Geometry check sheet. Reference: the model listing, model coordinates, mm. Round coordinates to 2 decimals unless told otherwise and drop trailing zeros. Order: outer loops, then holes, each group sorted by start corner. A loop starts at its lowest first (then second) coordinate and runs counter-clockwise, first axis right, second up. Notation, with made-up numbers: (-0.5, 47.5) - (20.5, 47.5) arc R30 ccw to (20.5, 79.5) - close; hole circle Ø7 at (-24, 49). An arc over 180 degrees is marked (long way). Use a Markdown table: item, result. Add a question column.
(1) Section check C-C on y = 1.05. Record the boundary of the cut face in (x, z).
(2) Gauge pin test, flat ends, axial feed: P1, Ø4.5, axis at x = 7.5, z = -7.5, coming from the +Y side; P2, Ø4.5, axis at x = 7.5, z = -78.5, coming from the -Y side; P3, Ø4, axis at x = 48.5, z = -7.5, coming from the +Y side. Record the tip position at first contact, or that the pin passes through.
(3) Section check A-A on x = 7.5. Record the boundary of the cut face in (y, z), then the cut area to 3 significant figures.
(4) Thickness scan on line 1 along X through (y, z) = (0.1, -7.5); line 2 along Z through (x, y) = (48.5, 0.1); line 3 along Z through (x, y) = (5.5, 0.9). Record the ranges inside material, lowest first. Write a range as [from, to].
(5) Section check B-B on z = -7.5. Record the boundary of the cut face in (x, y), then the cut area to 3 significant figures.
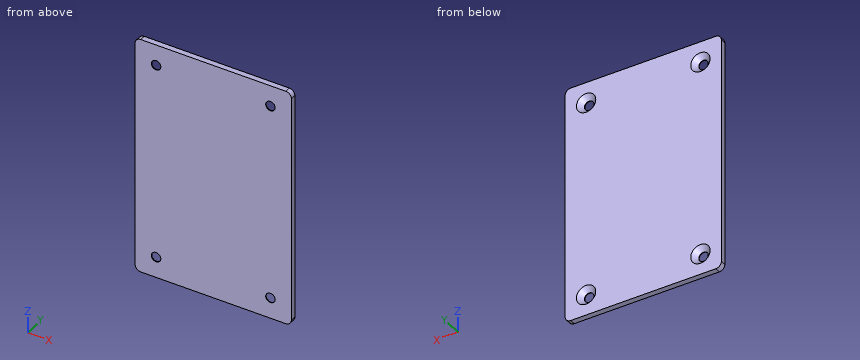
```python
from build123d import *

# Parameters (mm, degrees)
SKIZZE1_W                                   = 56
SKIZZE1_H                                   = 86
AUFSATZ_LINEAR_AUSTRAGEN1_DEPTH             = 2
VERRUNDUNG1_R                               = 2
FORMSENKUNG_F_R_M3_SENKSCHRAUBE_MIT_2_COUNT = 2
FORMSENKUNG_F_R_M3_SENKSCHRAUBE_MIT_2_PITCH = 81.987803971
FORMSENKUNG_F_R_M3_SENKSCHRAUBE_MIT_3_COUNT = 2
FORMSENKUNG_F_R_M3_SENKSCHRAUBE_MIT_3_PITCH = 71
FORMSENKUNG_F_R_M3_SENKSCHRAUBE_MIT_4_COUNT = 2
FORMSENKUNG_F_R_M3_SENKSCHRAUBE_MIT_4_PITCH = 41


with BuildPart() as part:
    # Skizze1 → Aufsatz-Linear austragen1 (new body)
    with BuildSketch(Plane(origin=(0, 0, 0), x_dir=(1, 0, 0), z_dir=(0, 1, 0))):
        with Locations((28, 43)):
            Rectangle(SKIZZE1_W, SKIZZE1_H)
    extrude(amount=AUFSATZ_LINEAR_AUSTRAGEN1_DEPTH)

    # Verrundung1
    verrundung1_edges = [part.edges().sort_by_distance(p)[0] for p in [
        (0, 1, -86),
        (56, 1, -86),
        (56, 1, 0),
        (0, 1, 0),
    ]]
    fillet(verrundung1_edges, radius=VERRUNDUNG1_R)

    # Skizze3 → Formsenkung für M3 Senkschraube mit Innensechskant1 (revolve, cut)
    with BuildSketch(Plane(origin=(7.5, 2, -7.5), x_dir=(0, 0, 1), z_dir=(1, 0, 0))):
        Polygon((0, 0), (0, 2), (1.7, 2), (1.7, 1.77), (3.47, 0), align=None)
    formsenkung_f_r_m3_senkschraube_mit_inne = revolve(axis=Axis((7.5, 8.35, -7.5), (0, -1, 0)), mode=Mode.SUBTRACT)

    # Formsenkung f_r M3 Senkschraube mit  2: Formsenkung für M3 Senkschraube mit Innensechskant1 ×2
    with Locations(*[Vector(0.5000743770922673, 0, -0.865982457891487) * (i * FORMSENKUNG_F_R_M3_SENKSCHRAUBE_MIT_2_PITCH) for i in range(1, FORMSENKUNG_F_R_M3_SENKSCHRAUBE_MIT_2_COUNT)]):
        add(formsenkung_f_r_m3_senkschraube_mit_inne, mode=Mode.SUBTRACT)

    # Formsenkung f_r M3 Senkschraube mit  3: Formsenkung für M3 Senkschraube mit Innensechskant1 ×2
    with Locations(*[(0, 0, -i * FORMSENKUNG_F_R_M3_SENKSCHRAUBE_MIT_3_PITCH) for i in range(1, FORMSENKUNG_F_R_M3_SENKSCHRAUBE_MIT_3_COUNT)]):
        add(formsenkung_f_r_m3_senkschraube_mit_inne, mode=Mode.SUBTRACT)

    # Formsenkung f_r M3 Senkschraube mit  4: Formsenkung für M3 Senkschraube mit Innensechskant1 ×2
    with Locations(*[(i * FORMSENKUNG_F_R_M3_SENKSCHRAUBE_MIT_4_PITCH, 0, 0) for i in range(1, FORMSENKUNG_F_R_M3_SENKSCHRAUBE_MIT_4_COUNT)]):
        add(formsenkung_f_r_m3_senkschraube_mit_inne, mode=Mode.SUBTRACT)


solid = part.part
```
Check sheet entries:
| question | item | result |
|---|---|---|
| 1 | outline | (0, -84) arc R2 ccw to (2, -86) - (54, -86) arc R2 ccw to (56, -84) - (56, -2) arc R2 ccw to (54, 0) - (2, 0) arc R2 ccw to (0, -2) - close; hole circle Ø5.04 at (7.5, -78.5); hole circle Ø5.04 at (7.5, -7.5); hole circle Ø5.04 at (48.5, -78.5); hole circle Ø5.04 at (48.5, -7.5) |
| 2 | P1 | stops at y = 0.78 |
| 2 | P2 | stops at y = 0 |
| 2 | P3 | stops at y = 0.53 |
| 3 | outline | (0, -86) - (2, -86) - (2, -81.97) - (0.23, -80.2) - (0, -80.2) - close; (0, -76.8) - (0.23, -76.8) - (2, -75.03) - (2, -10.97) - (0.23, -9.2) - (0, -9.2) - close; (0, -5.8) - (0.23, -5.8) - (2, -4.03) - (2, 0) - (0, 0) - close |
| 3 | area | 152 mm2 |
| 4 | line 1 | x = [0, 5.8], [9.2, 46.8], [50.2, 56] |
| 4 | line 2 | z = [-86, -80.2], [-76.8, -9.2], [-5.8, 0] |
| 4 | line 3 | z = [-86, -79.77], [-77.23, -8.77], [-6.23, 0] |
| 5 | outline | (0, 0) - (5.8, 0) - (5.8, 0.23) - (4.03, 2) - (0, 2) - close; (9.2, 0) - (46.8, 0) - (46.8, 0.23) - (45.03, 2) - (10.97, 2) - (9.2, 0.23) - close; (50.2, 0) - (56, 0) - (56, 2) - (51.97, 2) - (50.2, 0.23) - close |
| 5 | area | 92.1 mm2 |
